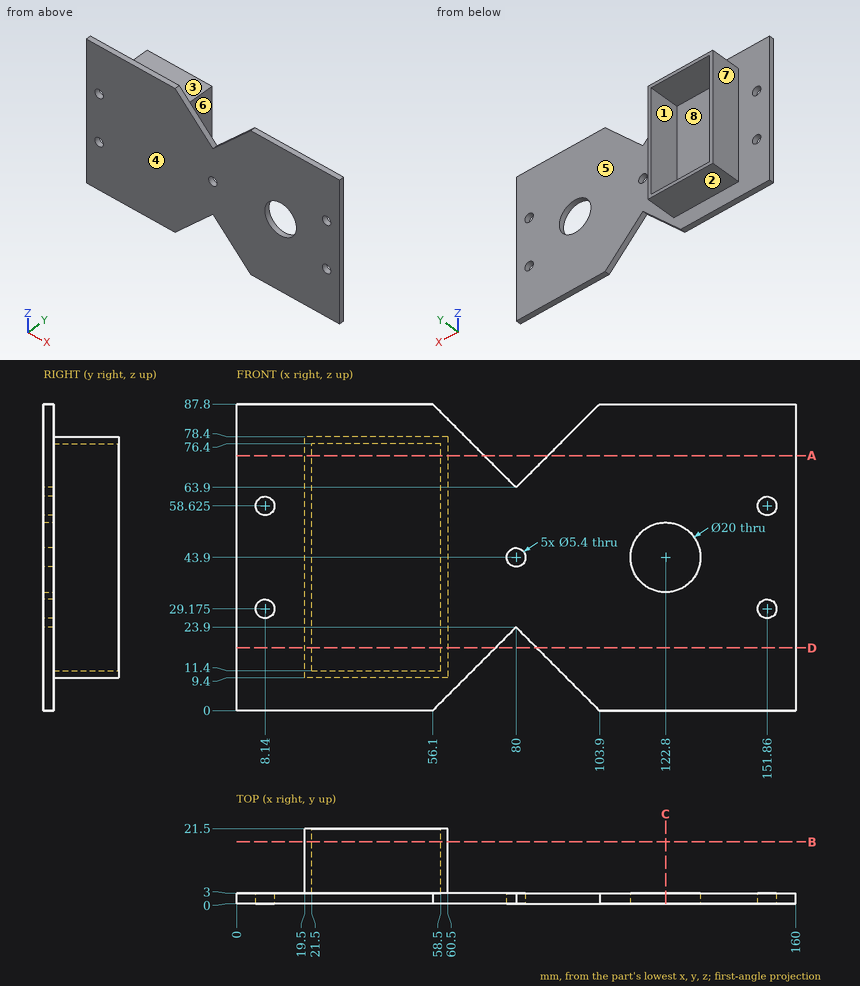
Design review of the part shown in the three views and the two pictorial views. Dimensions are in mm from the part's minimum x, y and z. A direction names the side the tool comes from. Coordinates: 2 decimals unless noted, no trailing zeros. Write each loop counter-clockwise with the first axis right and the second up, starting at its lowest first coordinate (ties: lowest second). Pieces come first, ordered by that corner, then holes. Notation, with made-up numbers: (16.5, 49) -> (60.5, 49) arc R18 ccw to (60.5, 58) -> close; hole circle Ø4 at (21, 26). An arc over 180 degrees is marked (long way). Answer in a Markdown table with one row per item.
1. Wall thickness on probe 1 along X at (y, z) = (7.25, 74.5); probe 2 along X at (y, z) = (2.5, 44); probe 3 along Y at (x, z) = (72, 34): over which ranges is each line inside the solid? List them lowest first. Write a range as [from, to].
Answers below:
| item | result |
|---|---|
| probe 1 | x = [19.5, 21.5], [58.5, 60.5] |
| probe 2 | x = [0, 77.3], [82.7, 112.8], [132.8, 160] |
| probe 3 | y = [0, 3] |
2. We need section B-B, the plane y = 17.75. State the section outline as (x, z) points.
Answers below:
| item | result |
|---|---|
| outline | (19.5, 9.4) -> (60.5, 9.4) -> (60.5, 78.4) -> (19.5, 78.4) -> close; hole (21.5, 11.4) -> (58.5, 11.4) -> (58.5, 76.4) -> (21.5, 76.4) -> close |
3. We need section A-A, the plane z = 73. State the section outline as (x, y) points.
Answers below:
| item | result |
|---|---|
| outline | (0, 0) -> (70.9, 0) -> (70.9, 3) -> (60.5, 3) -> (60.5, 21.5) -> (58.5, 21.5) -> (58.5, 3) -> (21.5, 3) -> (21.5, 21.5) -> (19.5, 21.5) -> (19.5, 3) -> (0, 3) -> close; (89.1, 0) -> (160, 0) -> (160, 3) -> (89.1, 3) -> close |
4. We need section C-C, the plane x = 122.8. State the section outline as (y, z) points, and give its area (3 significant figures).
Answers below:
| item | result |
|---|---|
| outline | (0, 0) -> (3, 0) -> (3, 33.9) -> (0, 33.9) -> close; (0, 53.9) -> (3, 53.9) -> (3, 87.8) -> (0, 87.8) -> close |
| area | 203 mm^2 |
5. We need section D-D, the plane z = 18. State the section outline as (x, y) points.
Answers below:
| item | result |
|---|---|
| outline | (0, 0) -> (74.1, 0) -> (74.1, 3) -> (60.5, 3) -> (60.5, 21.5) -> (58.5, 21.5) -> (58.5, 3) -> (21.5, 3) -> (21.5, 21.5) -> (19.5, 21.5) -> (19.5, 3) -> (0, 3) -> close; (85.9, 0) -> (160, 0) -> (160, 3) -> (85.9, 3) -> close |
6. Clearance check with flat-ended pins moving along their axes: pin 1 Ø10 at (y, z) = (18, 67.5) entering from +X; pin 2 Ø3 at (x, z) = (68.5, 10) entering from +Y; pin 3 Ø5.5 at (x, y) = (35.5, 14.5) entering from -Z; pin 4 Ø6 at (x, z) = (80, 43.9) entering from +Y. State where each tip first meets the part, or that it passes through.
Answers below:
| item | result |
|---|---|
| pin 1 | stops at x = 60.5 |
| pin 2 | passes through |
| pin 3 | stops at z = 9.4 |
| pin 4 | stops at y = 3 |
7. Draft analysis for pull direction X (two halves, no side actions). For the marked faces 5, 6, 7 and 8, state which applies: +X half, -X half, draft (parallel to the pull), parting line (faces both ways), or undercut.
Answers below:
| item | result |
|---|---|
| face 5 | draft |
| face 6 | +X half |
| face 7 | -X half |
| face 8 | undercut |
8. For the marked faces 1, 2, 3 and 4, list the 3-axis set-ups (+Z, -Z, +X, -X, +Y, -Y) from which the entire face can be reached by the end or side of a thin tool; tool diameter is ignored.
Answers below:
| item | result |
|---|---|
| face 1 | +Y |
| face 2 | -Z, +X, -X, +Y |
| face 3 | +Z, +X, -X, +Y |
| face 4 | +Z, -Z, +X, -X, -Y |
